from build123d import *

# Parameters (mm, degrees)
F0_W     = 2000
F0_H     = 1100
F1_DEPTH = 500
F2_W     = 350
F2_H     = 700
F3_DEPTH = 100
F4_R     = 25
F5_R     = 50


with BuildPart() as f1:
    # F0 (on Top) → F1 (new body)
    with BuildSketch(Plane.XY):
        with Locations((1000, 550)):
            Rectangle(F0_W, F0_H)
    extrude(amount=F1_DEPTH)

    # F2 (on face) → F3 (join)
    with BuildSketch(Plane.XY.offset(500)):
        with Locations((225, 550)):
            Rectangle(F2_W, F2_H)
    extrude(amount=F3_DEPTH)

    # F4
    f4_edges = [f1.edges().sort_by_distance(p)[0] for p in [
        (225, 200, 600),
        (50, 550, 600),
        (400, 550, 600),
        (225, 900, 600),
    ]]
    fillet(f4_edges, radius=F4_R)

    # F5
    f5_edges = [f1.edges().sort_by_distance(p)[0] for p in [
        (1000, 0, 500),
        (2000, 550, 500),
        (1000, 1100, 500),
    ]]
    fillet(f5_edges, radius=F5_R)


solid = f1.part
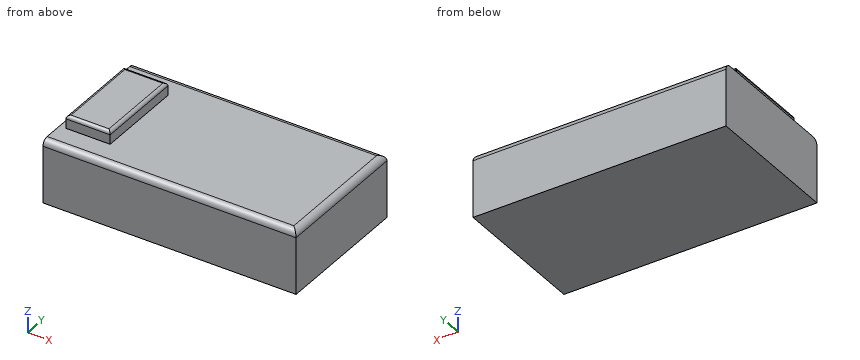
Geometry: final body of the model. Coordinates: model frame, mm. Coordinates: 2 decimals unless noted, no trailing zeros. Order: outer loops, then holes, each group sorted by start corner. A loop starts at its lowest first (then second) coordinate and runs counter-clockwise, first axis right, second up. Notation, with made-up numbers: M 11.25,-37 L 58.25,-37 A20 cw 58.25,-32 Z; hole C 52,-37 d9. An arc over 180 degrees is marked long. One line per question, with ' | ' between items. Start each with the question number.
Item 1: Ray query, probe 1 along Z at (x, y) = (1726.5, 1049); probe 2 along X at (y, z) = (508, 556). Return the intervals inside material, ascending. Write a range as [from, to].
Item 2: Cut plane C-C, the plane y = 112.5. Return the cut outline in (x, z).
Item 3: Cut plane B-B, the plane x = 782. Return the cut outline in (y, z), then the cut area to 3 significant figures.
Item 4: Pin query (flat end, axial travel): pin 1 Ø1 at (x, y) = (1413, 436.5) entering from +Z; pin 2 Ø12 at (x, z) = (1051.5, 460) entering from -Y; pin 3 Ø22.5 at (y, z) = (585.5, 521) entering from +X. Return the tip coordinate at first contact, or that it passes through.
Item 5: Cut plane A-A, the plane y = 753. Return the cut outline in (x, z).
A:
1) probe 1: z = [0, 500] | probe 2: x = [50, 400]
2) outline: M 0,0 L 2000,0 L 2000,450 A50 ccw 1950,500 L 0,500 Z
3) outline: M 0,0 L 1100,0 L 1100,450 A50 ccw 1050,500 L 50,500 A50 ccw 0,450 Z | area: 549,000 mm2
4) pin 1: stops at z = 500 | pin 2: stops at y = 0.16 | pin 3: stops at x = 400
5) outline: M 0,0 L 2000,0 L 2000,450 A50 ccw 1950,500 L 400,500 L 400,575 A25 ccw 375,600 L 75,600 A25 ccw 50,575 L 50,500 L 0,500 Z
